```python
from build123d import *

# Parameters (mm, degrees)
F0_W     = 7.62
F0_H     = 48.62068
F1_DEPTH = 5.08
F4_D     = 7.239
F5_D     = 7.239


with BuildPart() as f1:
    # F0 (on Front) → F1 (new body)
    with BuildSketch(Plane.XZ):
        with Locations((-3.7611387034, 15.5314761981)):
            Rectangle(F0_W, F0_H)
    extrude(amount=F1_DEPTH)

    # F4 (through all)
    with Locations(Plane.XZ.offset(5.08)):
        with Locations((-3.7611387034, 33.4918161981)):
            Hole(F4_D / 2)

    # F5 (through all)
    with Locations(Plane(origin=(0, 0, 0), x_dir=(1, 0, 0), z_dir=(0, 1, 0))):
        with Locations((-3.7611387034, 2.4288638019)):
            Hole(F5_D / 2)


solid = f1.part
```
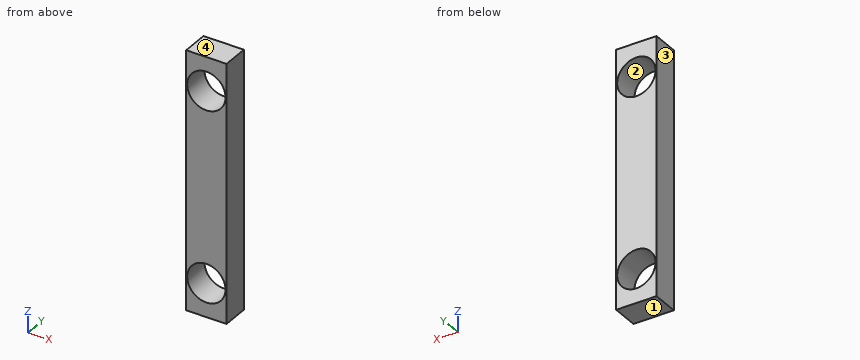
Part model, mm, in its own coordinate system. Face numbers are marked on the shaded views. Coordinates: 2 decimals unless noted, no trailing zeros. Write each loop counter-clockwise with the first axis right and the second up, starting at its lowest first coordinate (ties: lowest second). Pieces come first, ordered by that corner, then holes.
Item 1: Mould opens along Z. For the marked faces 1, 2, 3 and 4 say: released by +Z, released by -Z, zero draft, split by the parting line, or undercut.
Item 2: Slice it at D-D (x = -2). Write the cut outline in (y, z), and give its area (3 significant figures).
Item 3: Slice it at A-A (x = -4.5). Write the cut outline in (y, z).
Item 4: Pin check, flat tip, straight feed: pin 1 (1.5 mm diameter, centred on x = -2, z = -2.5, fed in from +Y). Stop position of the tip, or through.
Item 5: Slice it at B-B (z = 31). Write the cut outline in (x, y), and give its area (3 significant figures).
Item 6: Slice it at C-C (y = -2.8). Write the cut outline in (x, z), and give its area (3 significant figures).
Item 7: Probe line 1 (Z direction, x = -3.5, y = -3.85); line 2 (Z direction, x = -7, y = -0.9); line 3 (X direction, y = -2.45, z = -4). List the from-to ranges inside material, lowest first.
Results found:
1. face 1: released by -Z
1. face 2: undercut
1. face 3: zero draft
1. face 4: released by +Z
2. outline: (-5.08, -8.78) - (0, -8.78) - (0, -5.59) - (-5.08, -5.59) - close; (-5.08, 0.73) - (0, 0.73) - (0, 30.33) - (-5.08, 30.33) - close; (-5.08, 36.65) - (0, 36.65) - (0, 39.84) - (-5.08, 39.84) - close
2. area: 183 mm2
3. outline: (-5.08, -8.78) - (0, -8.78) - (0, -5.97) - (-5.08, -5.97) - close; (-5.08, 1.11) - (0, 1.11) - (0, 29.95) - (-5.08, 29.95) - close; (-5.08, 37.04) - (0, 37.04) - (0, 39.84) - (-5.08, 39.84) - close
4. pin 1: passes through
5. outline: (-7.57, -5.08) - (-6.39, -5.08) - (-6.39, 0) - (-7.57, 0) - close; (-1.14, -5.08) - (0.05, -5.08) - (0.05, 0) - (-1.14, 0) - close
5. area: 12.0 mm2
6. outline: (-7.57, -8.78) - (0.05, -8.78) - (0.05, 39.84) - (-7.57, 39.84) - close; hole circle Ø7.24 at (-3.76, -2.43); hole circle Ø7.24 at (-3.76, 33.49)
6. area: 288 mm2
7. line 1: z = -8.78 to -6.04, 1.18 to 29.88, 37.1 to 39.84
7. line 2: z = -8.78 to -4.04, -0.81 to 31.88, 35.11 to 39.84
7. line 3: x = -7.57 to -7.02, -0.5 to 0.05
